For this review, take the finished solid that the model builds, in its own axes (mm). Round coordinates to 2 decimals unless told otherwise and drop trailing zeros. Loops run counter-clockwise (first coordinate to the right, second up) from the corner with the lowest first, then second, coordinate; pieces in that order, holes last. Notation, with made-up numbers: (78.25, 9) -> (103.25, 9) arc R22 cw to (103.25, 15) -> close; hole circle Ø6 at (-29, 58.5). An arc over 180 degrees is marked (long way). Write each question's results on one line, items separated by ' | '.
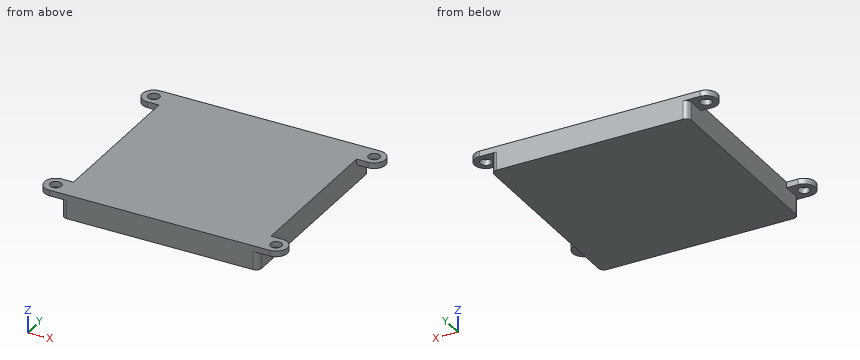
```python
from build123d import *

# Parameters (mm, degrees)
SKETCH1_W           = 70
SKETCH1_H           = 55
SKETCH1_R           = 2
BOSS_EXTRUDE1_DEPTH = 2
SKETCH2_W           = 70
SKETCH2_H           = 71
BOSS_EXTRUDE2_DEPTH = 6.5
FILLET1_R           = 2


with BuildPart() as part:
    # Sketch1 → Boss-Extrude1 (new body)
    # profile 1 of 3: a face of its own
    with BuildSketch(Plane.XY):
        Rectangle(SKETCH1_W, SKETCH1_H)
    # profile 2 of 3: a face of its own
    with BuildSketch(Plane.XY):
        with BuildLine():
            Line((-39, 27.5), (39, 27.5))
            ThreePointArc((39, 27.5), (43, 31.5), (39, 35.5))
            Line((39, 35.5), (-39, 35.5))
            ThreePointArc((-39, 35.5), (-43, 31.5), (-39, 27.5))
        make_face()
        with Locations((-39, 31.5)):
            Circle(SKETCH1_R, mode=Mode.SUBTRACT)
        with Locations((39, 31.5)):
            Circle(SKETCH1_R, mode=Mode.SUBTRACT)
    # profile 3 of 3: a face of its own
    with BuildSketch(Plane.XY):
        with BuildLine():
            ThreePointArc((39, -27.5), (43, -31.5), (39, -35.5))
            Line((39, -35.5), (-39, -35.5))
            ThreePointArc((-39, -35.5), (-43, -31.5), (-39, -27.5))
            Line((-39, -27.5), (39, -27.5))
        make_face()
        with Locations((-39, -31.5)):
            Circle(SKETCH1_R, mode=Mode.SUBTRACT)
        with Locations((39, -31.5)):
            Circle(SKETCH1_R, mode=Mode.SUBTRACT)
    extrude(amount=BOSS_EXTRUDE1_DEPTH)

    # Sketch2 → Boss-Extrude2 (add)
    with BuildSketch(Plane.XY):
        Rectangle(SKETCH2_W, SKETCH2_H)
    extrude(amount=-BOSS_EXTRUDE2_DEPTH)

    # Fillet1
    fillet1_edges = [part.edges().sort_by_distance(p)[0] for p in [
        (35, 35.5, -3.25),
        (35, -35.5, -3.25),
        (-35, -35.5, -3.25),
        (-35, 35.5, -3.25),
    ]]
    fillet(fillet1_edges, radius=FILLET1_R)


solid = part.part
```
1. For pin 1 (1.5 mm diameter, centred on y = 22.5, z = 0, fed in from -X); pin 2 (2.5 mm diameter, centred on y = 6.5, z = -1.5, fed in from +X); pin 3 (6.5 mm diameter, centred on x = 39, y = -31.5, fed in from -Z), all flat-tipped, find the tip position at first contact; note any pin that passes through.
Values found:
pin 1: stops at x = -35 | pin 2: stops at x = 35 | pin 3: stops at z = 0
2. Consider section C-C (y = -15.5). State the section outline as (x, z) points.
Values found:
outline: (-35, -6.5) -> (35, -6.5) -> (35, 2) -> (-35, 2) -> close
3. Consider section A-A (y = 31.5). State the section outline as (x, z) points.
Values found:
outline: (-43, 0) -> (-41, 0) -> (-41, 2) -> (-43, 2) -> close; (-37, 0) -> (-35, 0) -> (-35, -6.5) -> (35, -6.5) -> (35, 0) -> (37, 0) -> (37, 2) -> (-37, 2) -> close; (41, 0) -> (43, 0) -> (43, 2) -> (41, 2) -> close
4. Consider section B-B (z = -4). State the section outline as (x, y) points.
Values found:
outline: (-35, -33.5) arc R2 ccw to (-33, -35.5) -> (33, -35.5) arc R2 ccw to (35, -33.5) -> (35, 33.5) arc R2 ccw to (33, 35.5) -> (-33, 35.5) arc R2 ccw to (-35, 33.5) -> close
5. To check wall thickness, follow probe 1 along Y at (x, z) = (39, 1.5); probe 2 along X at (y, z) = (18, -5.75). State the ranges of each line that lie inside material, in increasing order.
Values found:
probe 1: y = -35.5 to -33.5, -29.5 to -27.5, 27.5 to 29.5, 33.5 to 35.5 | probe 2: x = -35 to 35
